The figure shows three views and two pictorial views of one solid part (mm, origin at its lowest corner). Answer the questions. A direction names the side the tool comes from. Give positions to 0.01 mm unless a question says otherwise; leave off trailing zeros. Loops run counter-clockwise (first coordinate to the right, second up) from the corner with the lowest first, then second, coordinate; pieces in that order, holes last. Notation, with made-up numbers: (88, 53) - (120, 53) arc R6 ccw to (120, 64) - close; hole circle Ø5 at (19, 31). An arc over 180 degrees is marked (long way). Use a Markdown table: item, result. Add a question column.
Item 1: For a pull along X with two mould halves and no side action, classify the marked faces 3 and 4 as +X half, -X half, draft (parallel to the pull), parting line (faces both ways), or undercut.
Item 2: Which of the six approach directions +Z, -Z, +X, -X, +Y, -Y give full straight-line access (tool end or side, diameter ignored) to the marked faces 1 and 2?
Item 3: A cutting plane is placed at A-A (y = 16). Determine the outline of the cut face in (x, z).
Item 4: Each of these flat-tipped pins is pushed along its axis until it touches: P1, Ø3, axis at x = 26, y = 8.5, coming from the -Z side; P2, Ø6, axis at x = 24, y = 13, coming from the +Z side. Where does it stop, or does it pass through?
Item 5: A cutting plane is placed at B-B (z = 3.5). Determine the outline of the cut face in (x, y), plus the area to 3 significant figures.
Item 6: A cutting plane is placed at C-C (z = 1.75). Determine the outline of the cut face in (x, y).
Item 7: Consider probe 1 along Y at (x, z) = (16, 6.1); probe 2 along Z at (x, y) = (16.5, 18); probe 3 along X at (y, z) = (19, 1). Determine where each line is inside the solid, lowest interval first. Write a range as [from, to].
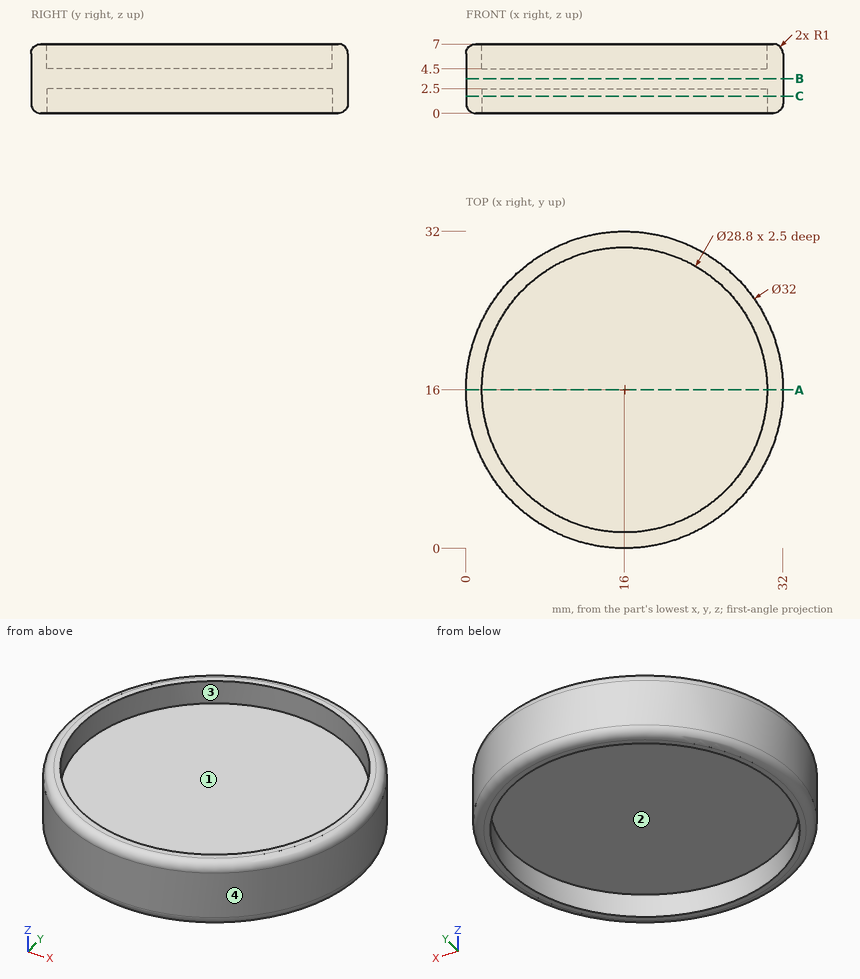
Geometry says:
| question | item | result |
|---|---|---|
| 1 | face 3 | undercut |
| 1 | face 4 | parting line |
| 2 | face 1 | +Z |
| 2 | face 2 | -Z |
| 3 | outline | (0, 1) arc R1 ccw to (1, 0) - (1.6, 0) - (1.6, 2.5) - (30.4, 2.5) - (30.4, 0) - (31, 0) arc R1 ccw to (32, 1) - (32, 6) arc R1 ccw to (31, 7) - (30.4, 7) - (30.4, 4.5) - (1.6, 4.5) - (1.6, 7) - (1, 7) arc R1 ccw to (0, 6) - close |
| 4 | P1 | z = 2.5 |
| 4 | P2 | z = 4.5 |
| 5 | outline | circle Ø32 at (16, 16) |
| 5 | area | 804 mm² |
| 6 | outline | circle Ø32 at (16, 16); hole circle Ø28.8 at (16, 16) |
| 7 | probe 1 | [0.01, 1.6], [30.4, 31.99] |
| 7 | probe 2 | [2.5, 4.5] |
| 7 | probe 3 | [0.28, 1.92], [30.08, 31.72] |
